Read the model definition and answer for the solid it produces. Units are mm, in the model's axes. Coordinates: 2 decimals unless noted, no trailing zeros. Loops run counter-clockwise (first coordinate to the right, second up) from the corner with the lowest first, then second, coordinate; pieces in that order, holes last. Notation, with made-up numbers: (17, 62.5) - (48, 62.5) arc R34 cw to (48, 101.5) - close; hole circle Ø1 at (-32, 63.25). An arc over 180 degrees is marked (long way). Use one line per item in the form item = value. Start each with the question number.
1) Each of these flat-tipped pins is pushed along its axis until it touches: P1, Ø1, axis at x = -33.5, z = 3.5, coming from the -Y side; P2, Ø5.5, axis at x = -31.75, y = 0, coming from the -Z side; P3, Ø2, axis at x = -16, z = 4.5, coming from the -Y side; P4, Ø3, axis at x = -10.5, y = 22, coming from the -Z side. Where does it stop, or does it pass through?
2) A cutting plane is placed at D-D (y = 27). Give the vertices of the cut face in (x, z) (3 decimals), and give its area (3 significant figures).
3) A cutting plane is placed at B-B (x = 0). Give the vertices of the cut face in (y, z) (1 decimal).
4) A cutting plane is placed at A-A (y = 0). Give the vertices of the cut face in (x, z) (1 decimal).
5) Consider line 1 (Z direction, x = -20, y = -43.5); line 2 (X direction, y = -32.5, z = 4.75); line 3 (Y direction, x = 31.75, z = 3.45) (3 decimals). Determine where each line is inside the solid, lowest interval first.
6) A cutting plane is placed at C-C (x = 31.75). Give the vertices of the cut face in (y, z) (3 decimals).
from build123d import *

# Parameters (mm, degrees)
SKETCH1_R           = 49.5046
BOSS_EXTRUDE1_DEPTH = 2.54
SKETCH2_R           = 47.6885
BOSS_EXTRUDE2_DEPTH = 3.175
SKETCH3_R           = 3.175
CUT_EXTRUDE1_DEPTH  = 6.715


with BuildPart() as part:
    # Sketch1 → Boss-Extrude1 (new body)
    with BuildSketch(Plane.XY):
        Circle(SKETCH1_R)
    extrude(amount=BOSS_EXTRUDE1_DEPTH)

    # Sketch2 → Boss-Extrude2 (add)
    with BuildSketch(Plane.XY.offset(2.54)):
        Circle(SKETCH2_R)
    extrude(amount=BOSS_EXTRUDE2_DEPTH)

    # Sketch3 → Cut-Extrude1 (cut, through all)
    with BuildSketch(Plane.XY.offset(5.715)):
        with Locations((-31.75, 0)):
            Circle(SKETCH3_R)
        with Locations((31.75, 0)):
            Circle(SKETCH3_R)
    extrude(amount=-CUT_EXTRUDE1_DEPTH, mode=Mode.SUBTRACT)


solid = part.part
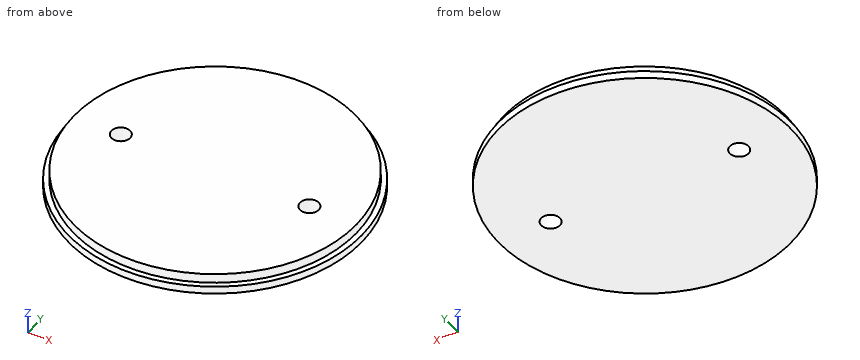
Found:
q1.P1 = -34.43
q1.P2 = through
q1.P3 = -45.27
q1.P4 = 0
q2.outline = (-41.493, 0) - (41.493, 0) - (41.493, 2.54) - (39.309, 2.54) - (39.309, 5.715) - (-39.309, 5.715) - (-39.309, 2.54) - (-41.493, 2.54) - close
q2.area = 460 mm^2
q3.outline = (-49.5, 0) - (49.5, 0) - (49.5, 2.5) - (47.7, 2.5) - (47.7, 5.7) - (-47.7, 5.7) - (-47.7, 2.5) - (-49.5, 2.5) - close
q4.outline = (-49.5, 0) - (-34.9, 0) - (-34.9, 5.7) - (-47.7, 5.7) - (-47.7, 2.5) - (-49.5, 2.5) - close; (-28.6, 0) - (28.6, 0) - (28.6, 5.7) - (-28.6, 5.7) - close; (34.9, 0) - (49.5, 0) - (49.5, 2.5) - (47.7, 2.5) - (47.7, 5.7) - (34.9, 5.7) - close
q5.line_1 = 0 to 2.54
q5.line_2 = -34.9 to 34.9
q5.line_3 = -35.583 to -3.175, 3.175 to 35.583
q6.outline = (-37.982, 0) - (-3.175, 0) - (-3.175, 5.715) - (-35.583, 5.715) - (-35.583, 2.54) - (-37.982, 2.54) - close; (3.175, 0) - (37.982, 0) - (37.982, 2.54) - (35.583, 2.54) - (35.583, 5.715) - (3.175, 5.715) - close
